Job drawing, mm, ordinate dimensions from the low corner. One solid piece. Round coordinates to 2 decimals unless told otherwise and drop trailing zeros. Loops run counter-clockwise (first coordinate to the right, second up) from the corner with the lowest first, then second, coordinate; pieces in that order, holes last. Notation, with made-up numbers: M -1,-35.75 L 41,-35.75 A21 ccw 41,-8.75 Z; hole C 4.5,46 d5. An arc over 180 degrees is marked long. Use a Markdown table: item, result. Add a question column.
(1) Wall check: L1, parallel to X at y = 2.9, z = 23; L2, parallel to X at y = 4.7, z = 9; L3, parallel to Y at x = 14.25, z = 20. Give the ranges that are in metal, low to high.
(2) Band-saw the part on B-B, the plane z = 17. Write the cut outline in (x, y).
(3) Band-saw the part on D-D, the plane y = 0.55. Write the cut outline in (x, z).
(4) Band-saw the part on C-C, the plane x = 2.8. Write the cut outline in (y, z), and give its area (3 significant figures).
(5) Flat gauge pins, fed straight in: P1, Ø2, axis at y = 4, z = 16.5, coming from the +X side; P2, Ø12, axis at x = 11, z = 36, coming from the -Y side; P3, Ø2.5, axis at y = 3, z = 6, coming from the +X side. Where does each tip first touch, or does it go through?
(6) Two-plate mould, pull along Y, no slides. Class the marked faces 1 and 2: released by +Y, released by -Y, zero draft, split by the parting line, or undercut.
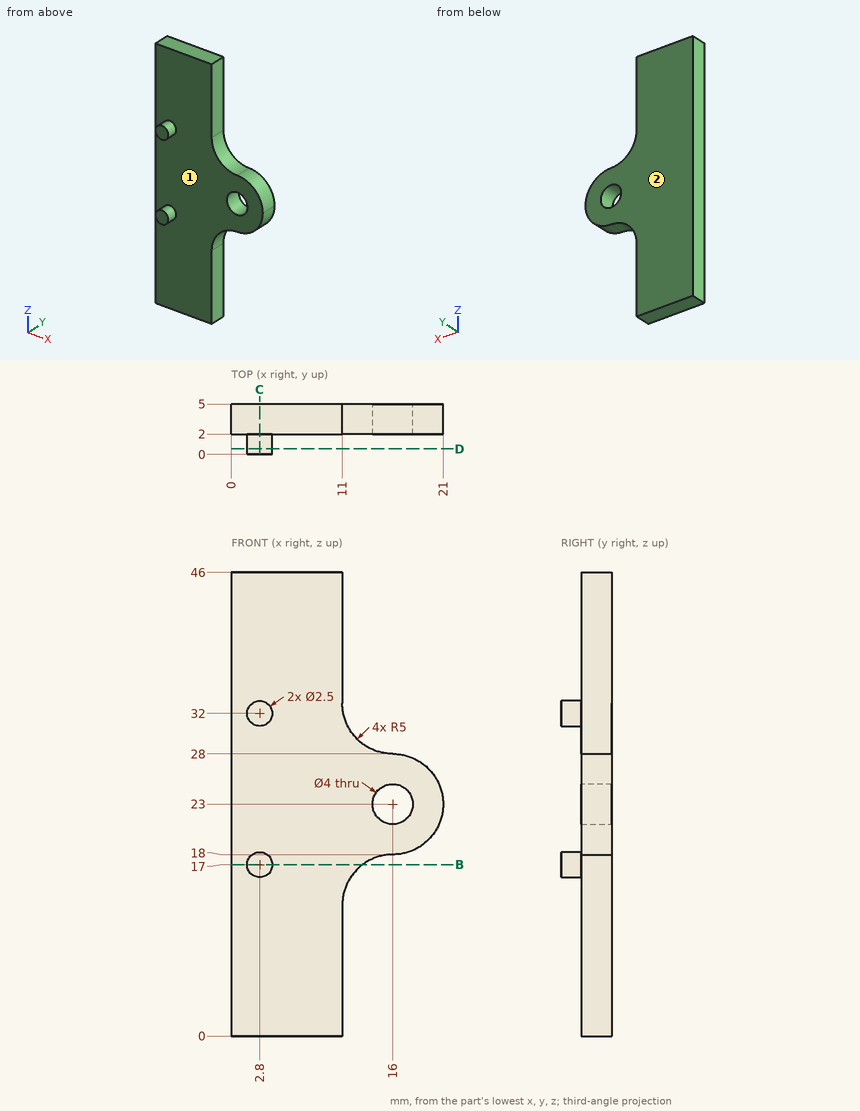
Return value:
| question | item | result |
|---|---|---|
| 1 | L1 | 0 to 14, 18 to 21 |
| 1 | L2 | 0 to 11 |
| 1 | L3 | 2 to 5 |
| 2 | outline | M 0,2 L 1.55,2 L 1.55,0 L 4.05,0 L 4.05,2 L 13,2 L 13,5 L 0,5 Z |
| 3 | outline | C 2.8,17 d2.5; C 2.8,32 d2.5 |
| 4 | outline | M 0,15.75 L 2,15.75 L 2,0 L 5,0 L 5,46 L 2,46 L 2,33.25 L 0,33.25 L 0,30.75 L 2,30.75 L 2,18.25 L 0,18.25 Z |
| 4 | area | 148 mm^2 |
| 5 | P1 | x = 13.82 |
| 5 | P2 | y = 2 |
| 5 | P3 | x = 11 |
| 6 | face 1 | released by -Y |
| 6 | face 2 | released by +Y |
